from build123d import *

# Parameters (mm, degrees)
FUEL_RING_SKETCH_W                = 6.7
FUEL_RING_SKETCH_H                = 2.5
CORE_MANIFOLD_SKETCH_W            = 6.7
CORE_MANIFOLD_SKETCH_H            = 1.6
FILM_MANIFOLD_SKETCH_W            = 2.8
FILM_MANIFOLD_SKETCH_H            = 1.5
PINTLE_SEAL_GROOVE_SKETCH_W       = 1.3
PINTLE_SEAL_GROOVE_SKETCH_H       = 2.4
FEED_PASSAGE_SKETCH_W             = 1.5
FEED_PASSAGE_SKETCH_H             = 48.905135707
FEED_PASSAGES_X3_COUNT            = 3
ETHANOL_HOLE_SKETCH_R             = 0.303840419
ETHANOL_HOLE_DEPTH                = 1.8
ETHANOL_HOLES_X8_COUNT            = 8
FILM_HOLE_SKETCH_R                = 0.333416852
FILM_HOLE_DEPTH                   = 1.8
FILM_HOLES_X8_COUNT               = 8
BOLT_HOLE_SKETCH_R                = 2.75
BOLT_HOLE_DEPTH                   = 9
BOLT_HOLES_X8_COUNT               = 8
IGNITER_PORT_4_ORB_SKETCH_R       = 4.953
IGNITER_PORT_4_ORB_DEPTH          = 10.5
IGNITER_PASSAGE_SKETCH_R          = 1.5
IGNITER_PASSAGE_DEPTH             = 22.5
PC_TAP_PORT_4_ORB_SKETCH_R        = 4.953
PC_TAP_PORT_4_ORB_DEPTH           = 10.5
PC_TAP_PASSAGE_SKETCH_R           = 0.75
PC_TAP_PASSAGE_DEPTH              = 22.5
ETHANOL_INLET_PORT_4_ORB_SKETCH_R = 4.953
ETHANOL_INLET_PORT_4_ORB_DEPTH    = 10.5
ETHANOL_INLET_PASSAGE_SKETCH_R    = 2
ETHANOL_INLET_PASSAGE_DEPTH       = 15.2
FILM_RESTRICTOR_SKETCH_R          = 0.434454496
FILM_RESTRICTOR_DEPTH             = 18.16
PINTLE_BOLT_TAP_DRILL_M4_SKETCH_R = 1.65
PINTLE_BOLT_TAP_DRILL_M4_DEPTH    = 10
PINTLE_BOLT_HOLES_X2_COUNT        = 2
TORCH_ETHANOL_PORT_SKETCH_R       = 3.5
TORCH_ETHANOL_PORT_DEPTH          = 8.6
TORCH_ETHANOL_DRILLING_SKETCH_R   = 1
TORCH_ETHANOL_DRILLING_DEPTH      = 15.2


with BuildPart() as part:
    # Body Sketch → Body (revolve)
    with BuildSketch(Plane.XY, mode=Mode.PRIVATE) as body_sk:
        Polygon((0, 9.594864293), (0, 82), (-9, 82), (-9, 68.2), (-22, 68.2), (-22, 9.594864293), align=None)
    revolve(body_sk.sketch.rotate(Axis((-60, 0, 0), (1, 0, 0)), 90), axis=Axis((-60, 0, 0), (1, 0, 0)))

    # Fuel Ring Sketch → Fuel Ring (revolve, cut)
    with BuildSketch(Plane.XY, mode=Mode.PRIVATE) as fuel_ring_sk:
        with Locations((-4.95, 59.9)):
            Rectangle(FUEL_RING_SKETCH_W, FUEL_RING_SKETCH_H)
    revolve(fuel_ring_sk.sketch.rotate(Axis((-60, 0, 0), (1, 0, 0)), 90), axis=Axis((-60, 0, 0), (1, 0, 0)), mode=Mode.SUBTRACT)

    # Core Manifold Sketch → Core Manifold (revolve, cut)
    with BuildSketch(Plane.XY, mode=Mode.PRIVATE) as core_manifold_sk:
        with Locations((-4.95, 10.994864293)):
            Rectangle(CORE_MANIFOLD_SKETCH_W, CORE_MANIFOLD_SKETCH_H)
    revolve(core_manifold_sk.sketch.rotate(Axis((-60, 0, 0), (1, 0, 0)), 90), axis=Axis((-60, 0, 0), (1, 0, 0)), mode=Mode.SUBTRACT)

    # Film Manifold Sketch → Film Manifold (revolve, cut)
    with BuildSketch(Plane.XY, mode=Mode.PRIVATE) as film_manifold_sk:
        with Locations((-3, 55.56918576)):
            Rectangle(FILM_MANIFOLD_SKETCH_W, FILM_MANIFOLD_SKETCH_H)
    revolve(film_manifold_sk.sketch.rotate(Axis((-60, 0, 0), (1, 0, 0)), 90), axis=Axis((-60, 0, 0), (1, 0, 0)), mode=Mode.SUBTRACT)

    # Pintle Seal Groove Sketch → Pintle Seal Groove (revolve, cut)
    with BuildSketch(Plane.XY, mode=Mode.PRIVATE) as pintle_seal_groove_sk:
        with Locations((-21.35, 12.4)):
            Rectangle(PINTLE_SEAL_GROOVE_SKETCH_W, PINTLE_SEAL_GROOVE_SKETCH_H)
    revolve(pintle_seal_groove_sk.sketch.rotate(Axis((-60, 0, 0), (1, 0, 0)), 90), axis=Axis((-60, 0, 0), (1, 0, 0)), mode=Mode.SUBTRACT)

    # Feed Passage Sketch → Feed Passage (revolve, cut)
    with BuildSketch(Plane.XY, mode=Mode.PRIVATE) as feed_passage_sk:
        with Locations((-6.05, 35.447432147)):
            Rectangle(FEED_PASSAGE_SKETCH_W, FEED_PASSAGE_SKETCH_H)
    feed_passage = revolve(feed_passage_sk.sketch.rotate(Axis((-6.8, 0, 0), (0, 1, 0)), 180), axis=Axis((-6.8, 0, 0), (0, 1, 0)), mode=Mode.SUBTRACT)

    # Feed Passages x3: Feed Passage ×3 about axis
    feed_passages_x3_axis = Axis((1.1, 0, 0), (-1, 0, 0))
    for i in range(1, FEED_PASSAGES_X3_COUNT):
        add(feed_passage.rotate(feed_passages_x3_axis, i * 360 / FEED_PASSAGES_X3_COUNT), mode=Mode.SUBTRACT)

    # Ethanol Hole Sketch → Ethanol Hole (cut)
    with BuildSketch(Plane(origin=(0, 0, 0), x_dir=(0, 0, -1), z_dir=(1, 0, 0))):
        with Locations((0, 10.598704712)):
            Circle(ETHANOL_HOLE_SKETCH_R)
    ethanol_hole = extrude(amount=-ETHANOL_HOLE_DEPTH, mode=Mode.SUBTRACT)

    # Ethanol Holes x8: Ethanol Hole ×8 about axis
    ethanol_holes_x8_axis = Axis((0, 0, 0), (1, 0, 0))
    for i in range(1, ETHANOL_HOLES_X8_COUNT):
        add(ethanol_hole.rotate(ethanol_holes_x8_axis, i * 360 / ETHANOL_HOLES_X8_COUNT), mode=Mode.SUBTRACT)

    # Film Hole Sketch → Film Hole (cut)
    with BuildSketch(Plane(origin=(0, 0, 0), x_dir=(0, 0, -1), z_dir=(1, 0, 0))):
        with Locations((21.26540674, 51.339233362)):
            Circle(FILM_HOLE_SKETCH_R)
    film_hole = extrude(amount=-FILM_HOLE_DEPTH, mode=Mode.SUBTRACT)

    # Film Holes x8: Film Hole ×8 about axis
    film_holes_x8_axis = Axis((0, 0, 0), (1, 0, 0))
    for i in range(1, FILM_HOLES_X8_COUNT):
        add(film_hole.rotate(film_holes_x8_axis, i * 360 / FILM_HOLES_X8_COUNT), mode=Mode.SUBTRACT)

    # Bolt Hole Sketch → Bolt Hole (cut)
    with BuildSketch(Plane(origin=(0, 0, 0), x_dir=(0, 0, -1), z_dir=(1, 0, 0))):
        with Locations((29.08394086, 70.214844471)):
            Circle(BOLT_HOLE_SKETCH_R)
    bolt_hole = extrude(amount=-BOLT_HOLE_DEPTH, mode=Mode.SUBTRACT)

    # Bolt Holes x8: Bolt Hole ×8 about axis
    bolt_holes_x8_axis = Axis((0, 0, 0), (1, 0, 0))
    for i in range(1, BOLT_HOLES_X8_COUNT):
        add(bolt_hole.rotate(bolt_holes_x8_axis, i * 360 / BOLT_HOLES_X8_COUNT), mode=Mode.SUBTRACT)

    # Igniter Port (-4 ORB) Sketch → Igniter Port (-4 ORB) (cut)
    with BuildSketch(Plane(origin=(-22, 0, 0), x_dir=(0, 0, -1), z_dir=(1, 0, 0))):
        with Locations(Location((0, -22.8, 0), (0, 0, 180))):
            Circle(IGNITER_PORT_4_ORB_SKETCH_R)
    extrude(amount=IGNITER_PORT_4_ORB_DEPTH, mode=Mode.SUBTRACT)

    # Igniter Passage Sketch → Igniter Passage (cut)
    with BuildSketch(Plane(origin=(-22, 0, 0), x_dir=(0, 0, -1), z_dir=(1, 0, 0))):
        with Locations(Location((0, -22.8, 0), (0, 0, 180))):
            Circle(IGNITER_PASSAGE_SKETCH_R)
    extrude(amount=IGNITER_PASSAGE_DEPTH, mode=Mode.SUBTRACT)

    # Pc Tap Port (-4 ORB) Sketch → Pc Tap Port (-4 ORB) (cut)
    with BuildSketch(Plane(origin=(-22, 0, 0), x_dir=(0, 0, -1), z_dir=(1, 0, 0))):
        with Locations(Location((16.943702021, -15.256177825, 0), (0, 0, 180))):
            Circle(PC_TAP_PORT_4_ORB_SKETCH_R)
    extrude(amount=PC_TAP_PORT_4_ORB_DEPTH, mode=Mode.SUBTRACT)

    # Pc Tap Passage Sketch → Pc Tap Passage (cut)
    with BuildSketch(Plane(origin=(-22, 0, 0), x_dir=(0, 0, -1), z_dir=(1, 0, 0))):
        with Locations(Location((16.943702021, -15.256177825, 0), (0, 0, 180))):
            Circle(PC_TAP_PASSAGE_SKETCH_R)
    extrude(amount=PC_TAP_PASSAGE_DEPTH, mode=Mode.SUBTRACT)

    # Ethanol Inlet Port (-4 ORB) Sketch → Ethanol Inlet Port (-4 ORB) (cut)
    with BuildSketch(Plane(origin=(-22, 0, 0), x_dir=(0, 0, -1), z_dir=(1, 0, 0))):
        with Locations(Location((0, 55.56918576, 0), (0, 0, 180))):
            Circle(ETHANOL_INLET_PORT_4_ORB_SKETCH_R)
    extrude(amount=ETHANOL_INLET_PORT_4_ORB_DEPTH, mode=Mode.SUBTRACT)

    # Ethanol Inlet Passage Sketch → Ethanol Inlet Passage (cut)
    with BuildSketch(Plane(origin=(-22, 0, 0), x_dir=(0, 0, -1), z_dir=(1, 0, 0))):
        with Locations(Location((0, 55.56918576, 0), (0, 0, 221.409622109))):
            Circle(ETHANOL_INLET_PASSAGE_SKETCH_R)
    extrude(amount=ETHANOL_INLET_PASSAGE_DEPTH, mode=Mode.SUBTRACT)

    # Film Restrictor Sketch → Film Restrictor (cut)
    with BuildSketch(Plane(origin=(-22, 0, 0), x_dir=(0, 0, -1), z_dir=(1, 0, 0))):
        with Locations(Location((0, 55.56918576, 0), (0, 0, 180))):
            Circle(FILM_RESTRICTOR_SKETCH_R)
    extrude(amount=FILM_RESTRICTOR_DEPTH, mode=Mode.SUBTRACT)

    # Pintle Bolt Tap Drill (M4) Sketch → Pintle Bolt Tap Drill (M4) (cut)
    with BuildSketch(Plane(origin=(-22, 0, 0), x_dir=(0, 0, -1), z_dir=(1, 0, 0))):
        with Locations((19, 0)):
            Circle(PINTLE_BOLT_TAP_DRILL_M4_SKETCH_R)
    pintle_bolt_tap_drill_m4 = extrude(amount=PINTLE_BOLT_TAP_DRILL_M4_DEPTH, mode=Mode.SUBTRACT)

    # Pintle Bolt Holes x2: Pintle Bolt Tap Drill (M4) ×2 about axis
    pintle_bolt_holes_x2_axis = Axis((0, 0, 0), (1, 0, 0))
    for i in range(1, PINTLE_BOLT_HOLES_X2_COUNT):
        add(pintle_bolt_tap_drill_m4.rotate(pintle_bolt_holes_x2_axis, i * 360 / PINTLE_BOLT_HOLES_X2_COUNT), mode=Mode.SUBTRACT)

    # Torch Ethanol Port Sketch → Torch Ethanol Port (cut)
    with BuildSketch(Plane(origin=(-22, 0, 0), x_dir=(0, 0, -1), z_dir=(1, 0, 0))):
        with Locations(Location((-22.516660498, -13, 0), (0, 0, 180))):
            Circle(TORCH_ETHANOL_PORT_SKETCH_R)
    extrude(amount=TORCH_ETHANOL_PORT_DEPTH, mode=Mode.SUBTRACT)

    # Torch Ethanol Drilling Sketch → Torch Ethanol Drilling (cut)
    with BuildSketch(Plane(origin=(-22, 0, 0), x_dir=(0, 0, -1), z_dir=(1, 0, 0))):
        with Locations(Location((-22.516660498, -13, 0), (0, 0, 180))):
            Circle(TORCH_ETHANOL_DRILLING_SKETCH_R)
    extrude(amount=TORCH_ETHANOL_DRILLING_DEPTH, mode=Mode.SUBTRACT)


solid = part.part
For this review, take the finished solid that the model builds, in its own axes (mm). A direction names the side the tool comes from. Round coordinates to 2 decimals unless told otherwise and drop trailing zeros. Loops run counter-clockwise (first coordinate to the right, second up) from the corner with the lowest first, then second, coordinate; pieces in that order, holes last. Notation, with made-up numbers: (-14.75, 16) - (1.25, 16) arc R19 cw to (1.25, 50) - close; hole circle Ø6 at (86, -11). An arc over 180 degrees is marked (long way). One line per item, written item: value. Start each with the question number.
Item 1: For L1, parallel to Y at x = -15.75, z = 0; L2, parallel to Y at x = -12.5, z = 0.5; L3, parallel to Z at x = -7.5, y = 45.5, list the stretches that pass through material, from the lowest coordinate up.
Item 2: For faces 5 (the cylindrical face through (-4.44, -28.49, -67.53)), 6 (the cylindrical face through (-2.98, -38.06, -41.51)), 7 (the flat face through (-11.5, -14, -17)), list the 3-axis set-ups (+Z, -Z, +X, -X, +Y, -Y) from which the entire face can be reached by the end or side of a thin tool; tool diameter is ignored.
Item 3: Take a section at C-C (z = 40.5). State how many separate pieces and enclosed holes the cut face has, plus the area to 3 significant figures.
Item 4: Take a section at A-A (y = 48). Give the boundary of the cut face in (x, z).
Item 5: Take a section at B-B (z = -65). Give the boundary of the cut face in (x, y).
Item 6: Clearance check with flat-ended pins moving along their axes: pin 1 Ø2.5 at (y, z) = (-22.8, 0) entering from -X; pin 2 Ø4 at (x, y) = (-17, 2) entering from -Z; pin 3 Ø2 at (x, z) = (-18, -2) entering from -Y; pin 4 Ø2 at (x, z) = (-6.5, 49) entering from -Y. State where each tip first meets the part, or that it passes through.
Item 7: The part is to be moulded in two halves that separate along Y. For faces 1 (the flat face through (0, -1, -17)), 2 (the cylindrical face through (-4.563, 31.406, 75.747)), 3 (the cylindrical face through (-4.4, 67.9, 27.6)), 4 (the flat face through (-1.6, -10, -3)), say which applies: +Y half, -Y half, draft (parallel to the pull), parting line (faces both ways), or undercut.
Answer below:
1. L1: y = -68.2 to -27.75, -17.85 to -9.59, 9.59 to 50.62, 60.52 to 68.2
1. L2: y = -68.2 to -27.73, -17.87 to -9.58, 9.58 to 50.64, 60.5 to 68.2
1. L3: z = -68.22 to -40.85, -37.01 to -1.33, 1.33 to 37.01, 40.85 to 68.22
2. face 5: +X, -X
2. face 6: none
2. face 7: -X
3. separate pieces: 1
3. enclosed holes: 5
3. area: 2,640 mm2
4. outline: (-22, -48.45) - (-9, -48.45) - (-9, -66.48) - (0, -66.48) - (0, 66.48) - (-9, 66.48) - (-9, 48.45) - (-22, 48.45) - close; hole (-8.3, -37.89) - (-1.6, -37.89) - (-1.6, -33.7) - (-8.3, -33.7) - close; hole circle Ø3 at (-6.8, 0); hole (-8.3, 33.7) - (-1.6, 33.7) - (-1.6, 37.89) - (-8.3, 37.89) - close; hole (-4.4, -29.46) - (-1.6, -29.46) - (-1.6, -26.48) - (-4.4, -26.48) - close; hole (-4.4, 26.48) - (-1.6, 26.48) - (-1.6, 29.46) - (-4.4, 29.46) - close
5. outline: (-22, -20.65) - (-9, -20.65) - (-9, -49.99) - (0, -49.99) - (0, 49.99) - (-9, 49.99) - (-9, 20.65) - (-22, 20.65) - close
6. pin 1: passes through
6. pin 2: stops at z = -68.2
6. pin 3: stops at y = -68.19
6. pin 4: stops at y = -66.48
7. face 1: draft
7. face 2: parting line
7. face 3: undercut
7. face 4: undercut
